Could you check a few things on this model? Use its own coordinates, in mm. Give positions to 0.01 mm unless a question says otherwise; leave off trailing zeros. Loops run counter-clockwise (first coordinate to the right, second up) from the corner with the lowest first, then second, coordinate; pieces in that order, holes last.
1. Imagine slicing it at A-A (x = 6.35). List the corners of the cut face in (y, z) for me (1 decimal).
2. Imagine slicing it at B-B (z = -6.35). Count the separate pieces of the cut face and the enclosed holes in it, plus the area to 3 significant figures.
3. Thinking about a two-plate mould opening in Z: for faces 1 (the cylindrical face through (4.01, 0.783, -8.496)), 2 (the flat face through (64, 1.588, -83)), 3 (the cylindrical face through (4.01, 0.783, -60.845)), which applies, +Z half, -Z half, draft (parallel to the pull), parting line (faces both ways), or undercut?
4. For P1, Ø4, axis at x = 123.82, z = -157.12, coming from the +Y side, with a flat end and sliding along its axis, tell me the tip position at first contact or that it passes through.
5. I need wall thicknesses on line 1 along X through (y, z) = (1.55, -56) (3 decimals); line 2 along X through (y, z) = (0.1, -56.5) (3 decimals). Which ranges of each line are inside material? Lowest first, please.
```python
from build123d import *

# Parameters (mm, degrees)
SKETCH1_W           = 130.175
SKETCH1_H           = 163.4744
SKETCH1_R           = 3.175
BOSS_EXTRUDE1_DEPTH = 1.5875


with BuildPart() as part:
    # Sketch1 → Boss-Extrude1 (new body)
    with BuildSketch(Plane(origin=(0, 0, 0), x_dir=(1, 0, 0), z_dir=(0, 1, 0))):
        with Locations((65.0875, 81.7372)):
            Rectangle(SKETCH1_W, SKETCH1_H)
        with Locations((6.35, 6.35)):
            Circle(SKETCH1_R, mode=Mode.SUBTRACT)
        with Locations((6.35, 157.1244)):
            Circle(SKETCH1_R, mode=Mode.SUBTRACT)
        with Locations((123.825, 6.35)):
            Circle(SKETCH1_R, mode=Mode.SUBTRACT)
        with Locations((123.825, 157.1244)):
            Circle(SKETCH1_R, mode=Mode.SUBTRACT)
        with Locations((6.35, 123.7869)):
            Circle(SKETCH1_R, mode=Mode.SUBTRACT)
        with Locations((6.35, 111.0869)):
            Circle(SKETCH1_R, mode=Mode.SUBTRACT)
        with Locations((6.35, 58.6994)):
            Circle(SKETCH1_R, mode=Mode.SUBTRACT)
        with Locations((6.35, 45.9994)):
            Circle(SKETCH1_R, mode=Mode.SUBTRACT)
        with Locations((123.825, 123.7869)):
            Circle(SKETCH1_R, mode=Mode.SUBTRACT)
        with Locations((123.825, 111.0869)):
            Circle(SKETCH1_R, mode=Mode.SUBTRACT)
        with Locations((123.825, 58.6994)):
            Circle(SKETCH1_R, mode=Mode.SUBTRACT)
        with Locations((123.825, 45.9994)):
            Circle(SKETCH1_R, mode=Mode.SUBTRACT)
    extrude(amount=BOSS_EXTRUDE1_DEPTH)


solid = part.part
```
Derived:
1. outline: (0, -163.5) - (1.6, -163.5) - (1.6, -160.3) - (0, -160.3) - close; (0, -153.9) - (1.6, -153.9) - (1.6, -127) - (0, -127) - close; (0, -120.6) - (1.6, -120.6) - (1.6, -114.3) - (0, -114.3) - close; (0, -107.9) - (1.6, -107.9) - (1.6, -61.9) - (0, -61.9) - close; (0, -55.5) - (1.6, -55.5) - (1.6, -49.2) - (0, -49.2) - close; (0, -42.8) - (1.6, -42.8) - (1.6, -9.5) - (0, -9.5) - close; (0, -3.2) - (1.6, -3.2) - (1.6, 0) - (0, 0) - close
2. separate pieces: 3
2. enclosed holes: 0
2. area: 186 mm2
3. face 1: undercut
3. face 2: draft
3. face 3: undercut
4. P1: passes through
5. line 1: x = 0 to 4.679, 8.021 to 122.154, 125.496 to 130.175
5. line 2: x = 0 to 4.06, 8.64 to 121.535, 126.115 to 130.175
